Here's the drawing with two shaded views (mm, measured from the low corner). I have some questions. A direction names the side the tool comes from. Give positions to 0.01 mm unless a question says otherwise; leave off trailing zeros. Loops run counter-clockwise (first coordinate to the right, second up) from the corner with the lowest first, then second, coordinate; pieces in that order, holes last. Notation, with made-up numbers: (-27.75, 1.5) -> (20.25, 1.5) arc R17 cw to (20.25, 17.5) -> close; hole circle Ø4 at (3.5, -15.75). An arc over 180 degrees is marked (long way). Answer in a Markdown table with one row per item. Add a question column.
Item 1: For P1, Ø6, axis at x = 105, y = 122.5, coming from the +Z side; P2, Ø5, axis at x = 251.5, y = 95.5, coming from the -Z side; P3, Ø7.5, axis at y = 160.5, z = 471.5, coming from the -X side, each with a flat end and sliding along its axis, tell me the tip position at first contact or that it passes through.
Item 2: If I drill on line 1 (X direction, y = 165.5, z = 227); line 2 (Z direction, x = 333, y = 144.5); line 3 (Y direction, x = 267, z = 1013), over which ranges is the centre line in solid material (lowest first)?
Item 3: If we section it at A-A (z = 114): Write out the boundary of the cut face in (x, y), then the cut area to 3 significant figures.
Item 4: If we section it at C-C (x = 163): Write out the boundary of the cut face in (y, z), then the cut area to 3 significant figures.
Item 5: Which directions (+Z, -Z, +X, -X, +Y, -Y) give clear straight access to the entire face, cutting with the end or side of a thin tool? Please do the marked faces 1, 2 and 3.
Item 6: If we section it at B-B (y = 93): Write out the boundary of the cut face in (x, z), then the cut area to 3 significant figures.
Item 7: If we section it at D-D (x = 34): Write out the boundary of the cut face in (y, z), then the cut area to 3 significant figures.
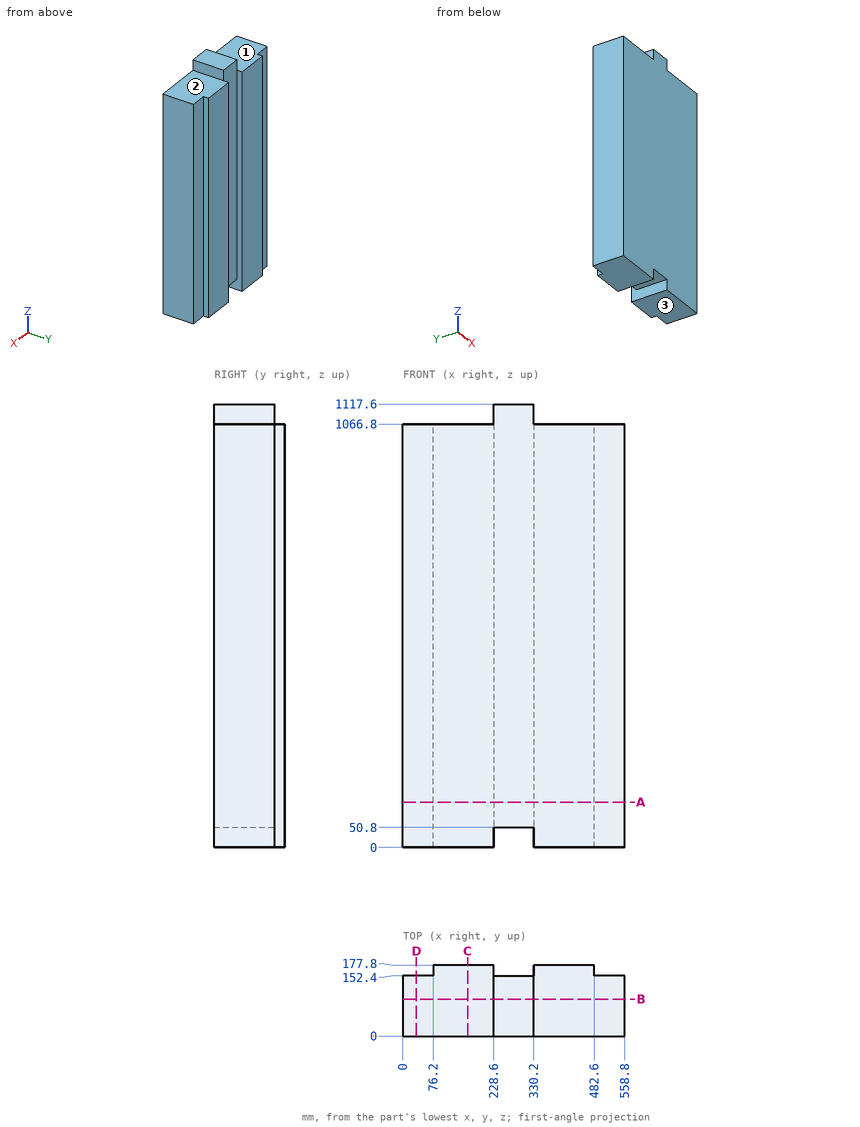
Recorded:
| question | item | result |
|---|---|---|
| 1 | P1 | stops at z = 1066.8 |
| 1 | P2 | stops at z = 50.8 |
| 1 | P3 | stops at x = 76.2 |
| 2 | line 1 | x = 76.2 to 228.6, 330.2 to 482.6 |
| 2 | line 2 | z = 0 to 1066.8 |
| 2 | line 3 | y = 0 to 152.4 |
| 3 | outline | (0, 0) -> (558.8, 0) -> (558.8, 152.4) -> (482.6, 152.4) -> (482.6, 177.8) -> (330.2, 177.8) -> (330.2, 152.4) -> (228.6, 152.4) -> (228.6, 177.8) -> (76.2, 177.8) -> (76.2, 152.4) -> (0, 152.4) -> close |
| 3 | area | 92,900 mm^2 |
| 4 | outline | (0, 0) -> (177.8, 0) -> (177.8, 1066.8) -> (0, 1066.8) -> close |
| 4 | area | 190,000 mm^2 |
| 5 | face 1 | +Z, -X, +Y, -Y |
| 5 | face 2 | +Z, +X, +Y, -Y |
| 5 | face 3 | -Z, +X, -X, +Y, -Y |
| 6 | outline | (0, 0) -> (228.6, 0) -> (228.6, 50.8) -> (330.2, 50.8) -> (330.2, 0) -> (558.8, 0) -> (558.8, 1066.8) -> (330.2, 1066.8) -> (330.2, 1117.6) -> (228.6, 1117.6) -> (228.6, 1066.8) -> (0, 1066.8) -> close |
| 6 | area | 596,000 mm^2 |
| 7 | outline | (0, 0) -> (152.4, 0) -> (152.4, 1066.8) -> (0, 1066.8) -> close |
| 7 | area | 163,000 mm^2 |
